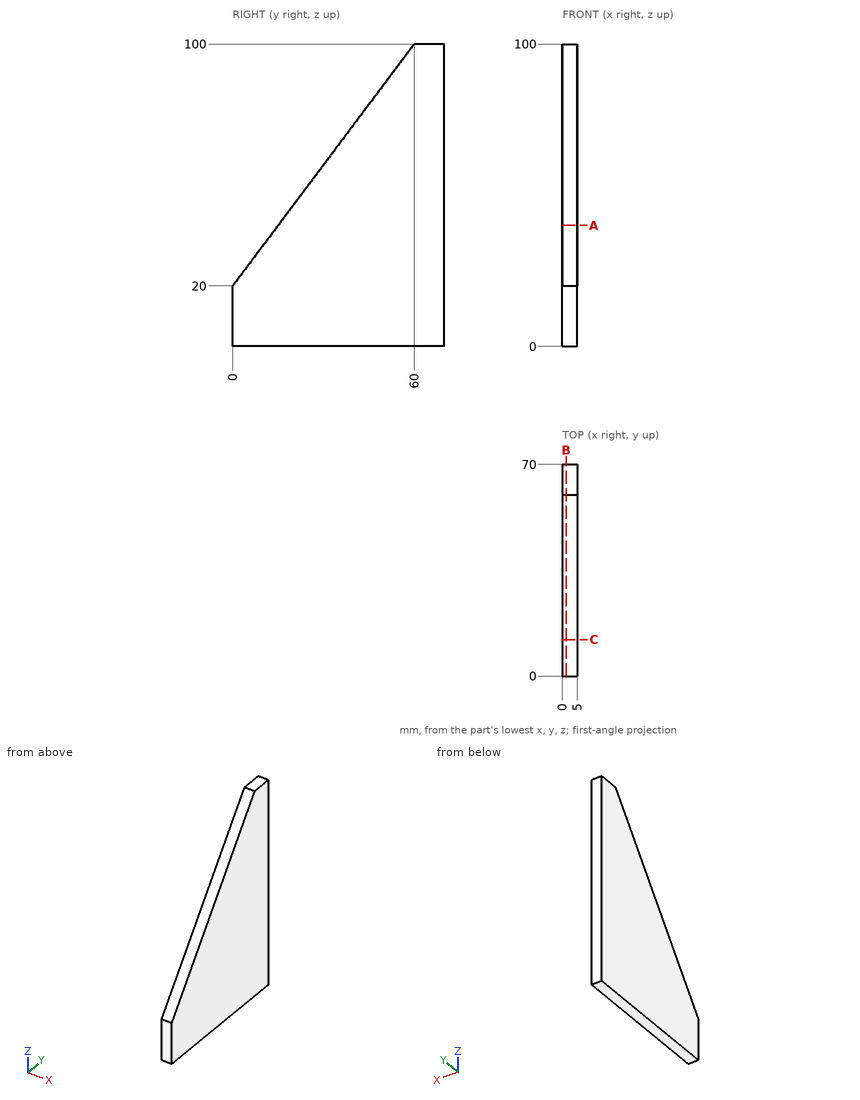
The drawing under review shows one solid part. Ordinate dimensions are in mm from its lowest x, y, z. Give positions to 0.01 mm unless a question says otherwise; leave off trailing zeros. Order: outer loops, then holes, each group sorted by start corner. A loop starts at its lowest first (then second) coordinate and runs counter-clockwise, first axis right, second up. Notation, with made-up numbers: (8.25, -3) - (30.25, -3) arc R19 cw to (30.25, 8) - close; hole circle Ø4 at (33.5, 53.5). An arc over 180 degrees is marked (long way). Answer as a JSON object with one key per item and string values. Group by question number.
Item 1: Take a section at A-A on z = 40. Give the boundary of the cut face in (x, y), and give its area (3 significant figures).
Item 2: Clearance check with a flat-ended pin moving along its axis: pin 1 Ø3 at (x, y) = (3, 27.5) entering from +Z. State where the tip first meets the part, or that it passes through.
Item 3: Take a section at B-B on x = 1.3. Give the boundary of the cut face in (y, z).
Item 4: Wall thickness on line 1 along Z through (x, y) = (0.8, 30); line 2 along Y through (x, z) = (4.15, 86); line 3 along Y through (x, z) = (2.8, 52.5) (3 decimals): over which ranges is each line inside the solid? List them lowest first.
Item 5: Take a section at C-C on y = 12. Give the boundary of the cut face in (x, z).
Reported:
{
 "1": {"outline": "(0, 15) - (5, 15) - (5, 70) - (0, 70) - close", "area": "275 mm^2"},
 "2": {"pin 1": "z = 58.67"},
 "3": {"outline": "(0, 0) - (70, 0) - (70, 100) - (60, 100) - (0, 20) - close"},
 "4": {"line 1": "0 to 60", "line 2": "49.5 to 70", "line 3": "24.375 to 70"},
 "5": {"outline": "(0, 0) - (5, 0) - (5, 36) - (0, 36) - close"}
}
